Geometry: final body of the model. Coordinates: model frame, mm. A direction names the side the tool comes from. Round coordinates to 2 decimals unless told otherwise and drop trailing zeros. Write each loop counter-clockwise with the first axis right and the second up, starting at its lowest first coordinate (ties: lowest second). Pieces come first, ordered by that corner, then holes. Notation, with made-up numbers: M 54,-14.5 L 58,-14.5 A29 ccw 58,14.5 Z; hole C -34.5,75.5 d6. An arc over 180 degrees is marked long. Put each result on its own line as item: value. Start each with the question number.
```python
from build123d import *

# Parameters (mm, degrees)
SKETCH1_R           = 100
SKETCH1_R_2         = 2.05
SKETCH1_R_3         = 63.5
BOSS_EXTRUDE1_DEPTH = 20
FILLET1_R           = 2
CUT_EXTRUDE1_START  = -10
CUT_EXTRUDE1_DEPTH  = 10
SKETCH3_R           = 2.525
CUT_EXTRUDE2_DEPTH  = 10


with BuildPart() as part:
    # Sketch1 → Boss-Extrude1 (new body)
    with BuildSketch(Plane(origin=(0, 0, 0), x_dir=(1, 0, 0), z_dir=(0, 1, 0))):
        with Locations(Location((0, 0, 0), (0, 0, 270))):
            Circle(SKETCH1_R)
        with Locations(Location((-78.5, 0, 0), (0, 0, 270))):
            Circle(SKETCH1_R_2, mode=Mode.SUBTRACT)
        with Locations(Location((0, 78.5, 0), (0, 0, 270))):
            Circle(SKETCH1_R_2, mode=Mode.SUBTRACT)
        with Locations(Location((78.5, 0, 0), (0, 0, 270))):
            Circle(SKETCH1_R_2, mode=Mode.SUBTRACT)
        with Locations(Location((0, -78.5, 0), (0, 0, 270))):
            Circle(SKETCH1_R_2, mode=Mode.SUBTRACT)
        with Locations(Location((0, 0, 0), (0, 0, 270))):
            Circle(SKETCH1_R_3, mode=Mode.SUBTRACT)
        with BuildLine():
            ThreePointArc((-27.60081718, 79.865166944), (-59.75052301, 59.75052301), (-79.865166944, 27.60081718))
            ThreePointArc((-79.865166944, 27.60081718), (-76.154088854, 19.970096414), (-68.523368088, 23.681174504))
            ThreePointArc((-68.523368088, 23.681174504), (-51.265241636, 51.265241636), (-23.681174504, 68.523368088))
            ThreePointArc((-23.681174504, 68.523368088), (-19.970096414, 76.154088854), (-27.60081718, 79.865166944))
        make_face(mode=Mode.SUBTRACT)
        with BuildLine():
            ThreePointArc((79.865166944, 27.60081718), (59.75052301, 59.75052301), (27.60081718, 79.865166944))
            ThreePointArc((27.60081718, 79.865166944), (19.970096414, 76.154088854), (23.681174504, 68.523368088))
            ThreePointArc((23.681174504, 68.523368088), (51.265241636, 51.265241636), (68.523368088, 23.681174504))
            ThreePointArc((68.523368088, 23.681174504), (76.154088854, 19.970096414), (79.865166944, 27.60081718))
        make_face(mode=Mode.SUBTRACT)
        with BuildLine():
            ThreePointArc((27.60081718, -79.865166944), (59.75052301, -59.75052301), (79.865166944, -27.60081718))
            ThreePointArc((79.865166944, -27.60081718), (76.154088854, -19.970096414), (68.523368088, -23.681174504))
            ThreePointArc((68.523368088, -23.681174504), (51.265241636, -51.265241636), (23.681174504, -68.523368088))
            ThreePointArc((23.681174504, -68.523368088), (19.970096414, -76.154088854), (27.60081718, -79.865166944))
        make_face(mode=Mode.SUBTRACT)
        with BuildLine():
            ThreePointArc((-79.865166944, -27.60081718), (-59.75052301, -59.75052301), (-27.60081718, -79.865166944))
            ThreePointArc((-27.60081718, -79.865166944), (-19.970096414, -76.154088854), (-23.681174504, -68.523368088))
            ThreePointArc((-23.681174504, -68.523368088), (-51.265241636, -51.265241636), (-68.523368088, -23.681174504))
            ThreePointArc((-68.523368088, -23.681174504), (-76.154088854, -19.970096414), (-79.865166944, -27.60081718))
        make_face(mode=Mode.SUBTRACT)
    extrude(amount=BOSS_EXTRUDE1_DEPTH)

    # Fillet1
    fillet1_edges = [part.edges().sort_by_distance(p)[0] for p in [
        (0, 0, -100),
        (0, 20, -100),
        (0, 0, -63.5),
        (0, 20, -63.5),
    ]]
    fillet(fillet1_edges, radius=FILLET1_R)

    # Sketch2 → Cut-Extrude1 (cut)
    with BuildSketch(Plane(origin=(0, 20, 0), x_dir=(1, 0, 0), z_dir=(0, 1, 0)).offset(CUT_EXTRUDE1_START)):
        with BuildLine():
            Line((-19.777543396, 75.467030422), (-24.444340717, 96.966356057))
            ThreePointArc((-24.444340717, 96.966356057), (-70.710678119, 70.710678119), (-96.966356057, 24.444340717))
            Line((-96.966356057, 24.444340717), (-75.467030422, 19.777543396))
            ThreePointArc((-75.467030422, 19.777543396), (-71.253946926, 20.410841463), (-68.523368088, 23.681174504))
            ThreePointArc((-68.523368088, 23.681174504), (-51.265241636, 51.265241636), (-23.681174504, 68.523368088))
            ThreePointArc((-23.681174504, 68.523368088), (-20.410841463, 71.253946926), (-19.777543396, 75.467030422))
        make_face()
        with BuildLine():
            Line((19.777543396, -75.467030422), (24.444340717, -96.966356057))
            ThreePointArc((24.444340717, -96.966356057), (70.710678119, -70.710678119), (96.966356057, -24.444340717))
            Line((96.966356057, -24.444340717), (75.467030422, -19.777543396))
            ThreePointArc((75.467030422, -19.777543396), (71.253946926, -20.410841463), (68.523368088, -23.681174504))
            ThreePointArc((68.523368088, -23.681174504), (51.265241636, -51.265241636), (23.681174504, -68.523368088))
            ThreePointArc((23.681174504, -68.523368088), (20.410841463, -71.253946926), (19.777543396, -75.467030422))
        make_face()
    extrude(amount=CUT_EXTRUDE1_DEPTH, mode=Mode.SUBTRACT)

    # Sketch3 → Cut-Extrude2 (cut)
    with BuildSketch(Plane(origin=(0, 10, 0), x_dir=(1, 0, 0), z_dir=(0, 1, 0))):
        with Locations(Location((-45.111909622, 80.467248681, 0), (0, 0, 270))):
            Circle(SKETCH3_R)
        with Locations(Location((-65.230600564, 65.230600564, 0), (0, 0, 270))):
            Circle(SKETCH3_R)
        with Locations(Location((-80.467248681, 45.111909622, 0), (0, 0, 270))):
            Circle(SKETCH3_R)
        with Locations(Location((45.111909622, -80.467248681, 0), (0, 0, 90))):
            Circle(SKETCH3_R)
        with Locations(Location((65.230600564, -65.230600564, 0), (0, 0, 90))):
            Circle(SKETCH3_R)
        with Locations(Location((80.467248681, -45.111909622, 0), (0, 0, 90))):
            Circle(SKETCH3_R)
    extrude(amount=-CUT_EXTRUDE2_DEPTH, mode=Mode.SUBTRACT)


solid = part.part
```
1) Ray query, probe 1 along X at (y, z) = (7.75, 0); probe 2 along X at (y, z) = (19.25, -28); probe 3 along Z at (x, y) = (28, 13.75). Return the intervals inside material, ascending.
2) Section B-B, the plane z = 31. Give the number of separate pieces and of enclosed holes in the cut face, and give its area (3 significant figures).
3) Draft query along Z for faces 1 (the face through (-86.367, 14.93, -22.144)), 2 (the face through (59, 20, -29)), 3 (the face through (-20.015, 9.86, 76.278)). Return one class per face: +Z half, -Z half, draft (parallel to the pull), parting line (faces both ways), or undercut.
4) Section A-A, the plane y = 14. Output: boundary loops of the cut face in (x, z), and give its area (3 significant figures).
5) First-contact query: pin 1 (10 mm diameter, centred on y = 14, z = 17, fed in from +X); pin 2 (10 mm diameter, centred on y = 10, z = 21, fed in from -X); pin 3 (2 mm diameter, centred on y = 4.5, z = 53, fed in from -X). Flat tips, straight axial feed; report the tip coordinate or a pass-through.
6) Access query for faces 4 (the face through (-50.94, 9.86, 51.59)), 5 (the face through (0, 0, -66)), 6 (the face through (22.08, 14.93, 86.07)), 7 (the face through (86.367, 14.93, 22.144)). Directions: +Z, -Z, +X, -X, +Y, -Y. A direction counts if a zero-diameter tool reaches every point of the face in a straight line with its end or side. Return the directions, or none.
Solved:
1. probe 1: x = -100 to -80.55, -76.45 to -63.5, 63.5 to 76.45, 80.55 to 100
1. probe 2: x = -66.87 to -57.48, 57.48 to 66.87, 79.73 to 95.54
1. probe 3: z = -96 to -79.73, -66.87 to -56.99, 56.99 to 66.87
2. separate pieces: 4
2. enclosed holes: 0
2. area: 892 mm2
3. face 1: -Z half
3. face 2: draft
3. face 3: undercut
4. outline: M -96.97,-24.44 L -75.47,-19.78 A6 cw -68.52,-23.68 A72.5 ccw -23.68,-68.52 A6 cw -19.78,-75.47 L -24.44,-96.97 A100 ccw 96.97,24.44 L 75.47,19.78 A6 cw 68.52,23.68 A72.5 ccw 23.68,68.52 A6 cw 19.78,75.47 L 24.44,96.97 A100 ccw Z; hole C -78.5,0 d4.1; hole M -79.87,27.6 A6 ccw -68.52,23.68 A72.5 cw -23.68,68.52 A6 ccw -27.6,79.87 A84.5 ccw Z; hole C 0,0 d127; hole C 0,-78.5 d4.1; hole C 0,78.5 d4.1; hole M 23.68,-68.52 A6 ccw 27.6,-79.87 A84.5 ccw 79.87,-27.6 A6 ccw 68.52,-23.68 A72.5 cw Z; hole C 78.5,0 d4.1
4. area: 11,700 mm2
5. pin 1: stops at x = 99.28
5. pin 2: stops at x = -98.71
5. pin 3: stops at x = -85.42
6. face 4: +Y, -Y
6. face 5: +Z, -Z, +X, -X, -Y
6. face 6: +X, +Y
6. face 7: +Z, +Y
